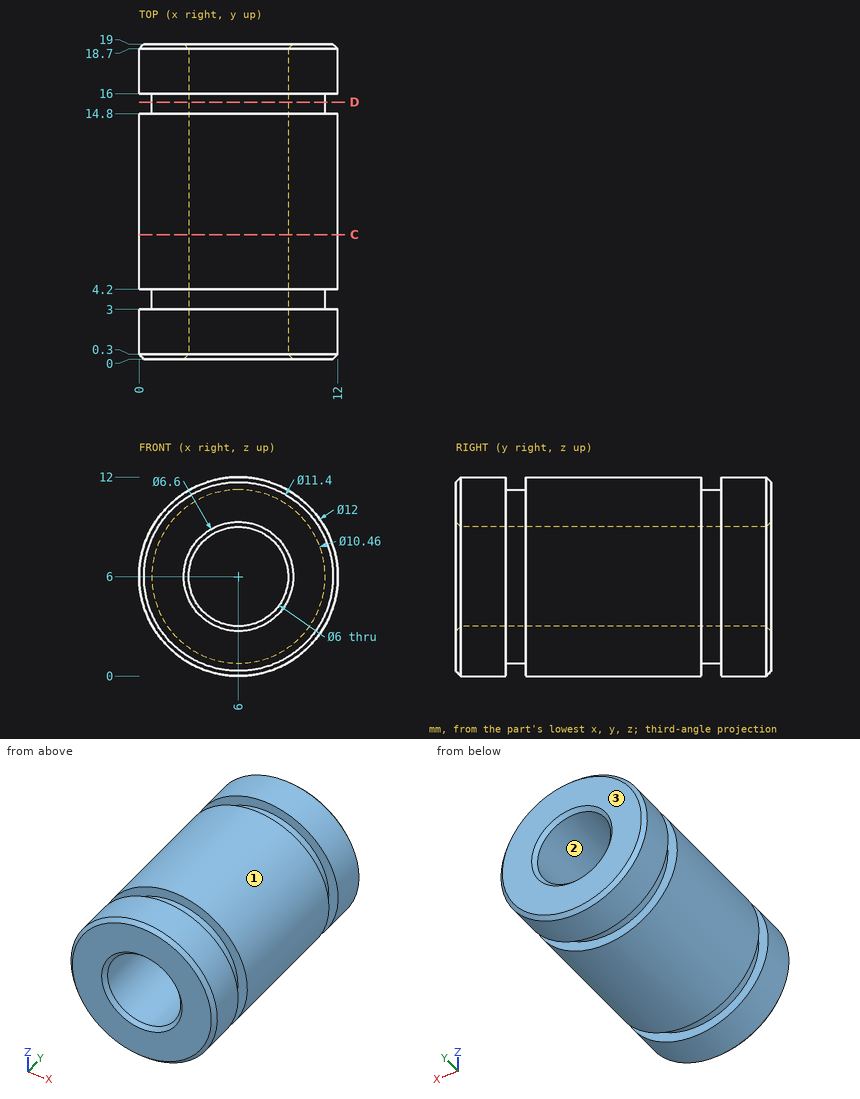
Study the drawing (mm; zero at the part's minimum x, y, z) and answer. Give positions to 0.01 mm unless a question says otherwise; leave off trailing zeros. Order: outer loops, then holes, each group sorted by start corner. A loop starts at its lowest first (then second) coordinate and runs counter-clockwise, first axis right, second up.
1. Section D-D, the plane y = 15.5 is taken. Determine the outline of the cut face in (x, z).
Result sheet:
outline: circle Ø10.46 at (6, 6); hole circle Ø6 at (6, 6)
2. Straight lines are drawn through the part: L1, parallel to Y at x = 10.5, z = 9.25; L2, parallel to X at y = 11, z = 6; L3, parallel to X at y = 13, z = 8.5. For each, find the intervals that lie inside material, in ascending order.
Result sheet:
L1: y = 0 to 3, 4.2 to 14.8, 16 to 19
L2: x = 0 to 3, 9 to 12
L3: x = 0.55 to 4.34, 7.66 to 11.45
3. Section C-C, the plane y = 7.5 is taken. Determine the outline of the cut face in (x, z).
Result sheet:
outline: circle Ø12 at (6, 6); hole circle Ø6 at (6, 6)
4. Each of these flat-tipped pins is pushed along its axis until it touches: P1, Ø2, axis at y = 11, z = 6.5, coming from the -X side; P2, Ø2, axis at y = 12.5, z = 9.5, coming from the +X side; P3, Ø1.5, axis at x = 7, y = 9, coming from the +Z side. Where does it stop, or does it pass through?
Result sheet:
P1: stops at x = 0
P2: stops at x = 11.45
P3: stops at z = 11.99
5. The mould has two halves that part along X. Classify the marked faces 1, 2 and 3: released by +X, released by -X, zero draft, split by the parting line, or undercut.
Result sheet:
face 1: split by the parting line
face 2: undercut
face 3: zero draft
